The listing builds one solid part. Answer for the finished solid, in the listing's coordinates (mm). Face numbers are marked on the shaded views. Give positions to 0.01 mm unless a question says otherwise; leave off trailing zeros. Loops run counter-clockwise (first coordinate to the right, second up) from the corner with the lowest first, then second, coordinate; pieces in that order, holes last. Notation, with made-up numbers: M 5,26 L 60,26 A21 cw 60,52 Z; hole C 76.5,3 d7. An arc over 180 degrees is marked long. Use one line per item in the form item = value. Start each with the question number.
1. The part is cut by section A-A (x = 0). Write down the section's boundary in (y, z), and give its area (3 significant figures).
2. The part is cut by section D-D (z = 59). Write down the section's boundary in (x, y).
3. The mould has two halves that part along X. Classify the marked faces 1, 2 and 3: released by +X, released by -X, zero draft, split by the parting line, or undercut.
4. Straight lines are drawn through the part: line 1 (Y direction, x = 0, z = 33); line 2 (Y direction, x = -4, z = 40); line 3 (X direction, y = -2.5, z = 52.5). For each, find the intervals that lie inside material, in ascending order. Write a range as from..to.
5. The part is cut by section C-C (z = 16.5). Write down the section's boundary in (x, y).
6. Each of these flat-tipped pins is pushed along its axis until it touches: pin 1 Ø6 at (x, z) = (-5.5, 40) entering from -Y; pin 2 Ø12 at (y, z) = (3.5, 51.5) entering from -X; pin 3 Ø5 at (y, z) = (8, 46) entering from +X; pin 4 Ø8 at (x, z) = (9, 42.5) entering from +Y. Where does it stop, or does it pass through?
from build123d import *

# Parameters (mm, degrees)
SKETCH1_R           = 16.7
SKETCH1_R_2         = 12.15
BOSS_EXTRUDE1_DEPTH = 70


# Read off the part's stored shape, not the designer's step: M33x3.5 Machine Threads Stud1
with BuildPart() as part:
    # Sketch1 → Boss-Extrude1 (new body)
    with BuildSketch(Plane.XY):
        Circle(SKETCH1_R)
        Circle(SKETCH1_R_2, mode=Mode.SUBTRACT)
    extrude(amount=BOSS_EXTRUDE1_DEPTH)

    # M33x3.5 Machine Threads Stud1 outline → M33x3.5 Machine Threads Stud1 (revolve, cut)
    with BuildSketch(Plane.XZ):
        Polygon((14.579, 0), (16.7, 0), (16.7, 24), (16.5, 24), (16.5, 1.921), align=None)
    revolve(axis=Axis((0, 0, 0), (0, 0, 1)), mode=Mode.SUBTRACT)


solid = part.part
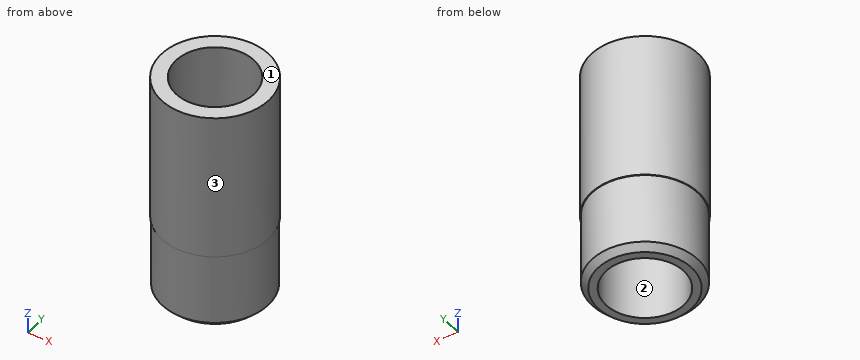
Derived:
q1.outline = M -16.7,24 L -16.5,24 L -16.5,1.92 L -14.58,0 L -12.15,0 L -12.15,70 L -16.7,70 Z; M 12.15,0 L 14.58,0 L 16.5,1.92 L 16.5,24 L 16.7,24 L 16.7,70 L 12.15,70 Z
q1.area = 624 mm2
q2.outline = C 0,0 d33.4; hole C 0,0 d24.3
q3.face_1 = zero draft
q3.face_2 = undercut
q3.face_3 = split by the parting line
q4.line_1 = -16.7..-12.15, 12.15..16.7
q4.line_2 = -16.21..-11.47, 11.47..16.21
q4.line_3 = -16.51..-11.89, 11.89..16.51
q5.outline = C 0,0 d33; hole C 0,0 d24.3
q6.pin_1 = -16.51
q6.pin_2 = -16.7
q6.pin_3 = 15.77
q6.pin_4 = 15.93
